Job drawing, mm, ordinate dimensions from the low corner. One solid piece. Give positions to 0.01 mm unless a question says otherwise; leave off trailing zeros. Order: outer loops, then holes, each group sorted by start corner. A loop starts at its lowest first (then second) coordinate and runs counter-clockwise, first axis right, second up.
1. Probe line 1 (Z direction, x = 76, y = 4); line 2 (X direction, y = 2.25, z = 102.5). List the from-to ranges inside material, lowest first.
2. Slice it at B-B on y = 4.5. List the corners of the cut face in (x, z).
3. Slice it at A-A on x = 91. List the corners of the cut face in (y, z), and give its area (3 significant figures).
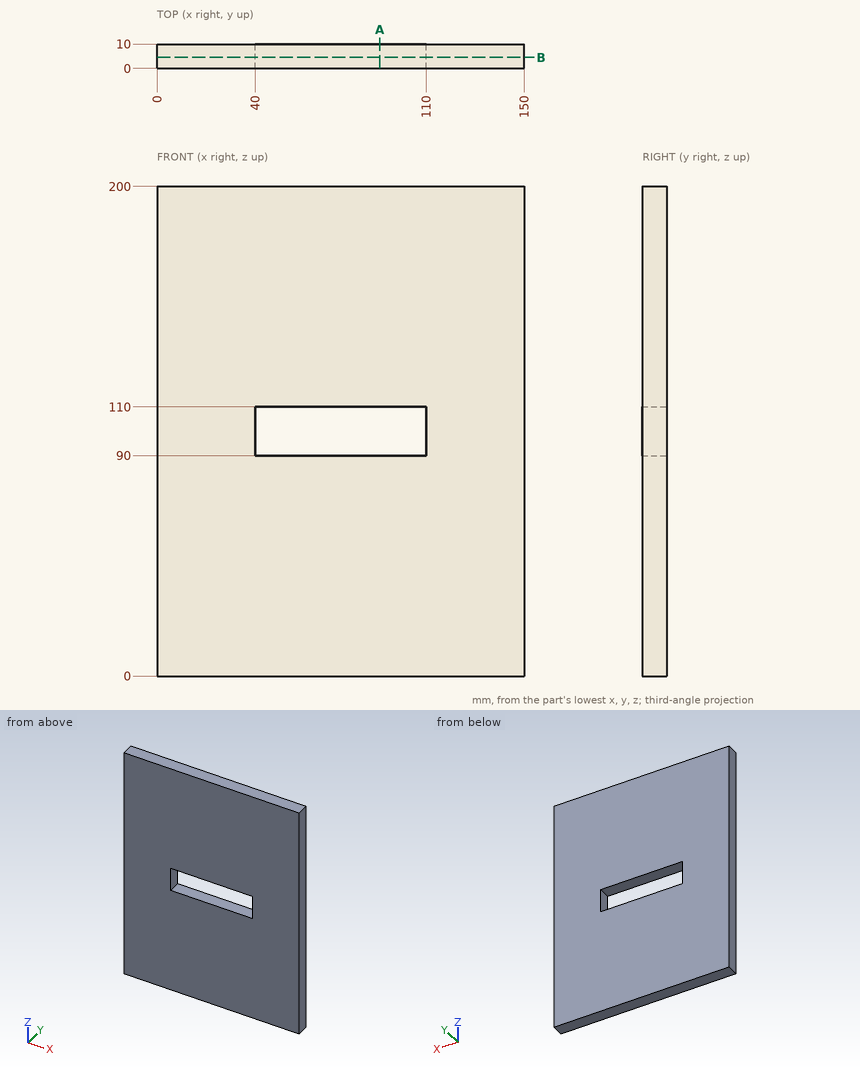
Data:
1. line 1: z = 0 to 90, 110 to 200
1. line 2: x = 0 to 40, 110 to 150
2. outline: (0, 0) - (150, 0) - (150, 200) - (0, 200) - close; hole (40, 90) - (110, 90) - (110, 110) - (40, 110) - close
3. outline: (0, 0) - (10, 0) - (10, 90) - (0, 90) - close; (0, 110) - (10, 110) - (10, 200) - (0, 200) - close
3. area: 1,800 mm2
